Source: CAD feature listing. Evaluate the final solid. Frame: model axes, mm. Face numbers are marked on the shaded views. A direction names the side the tool comes from. Give positions to 0.01 mm unless a question says otherwise; leave off trailing zeros. Write each loop counter-clockwise with the first axis right and the second up, starting at its lowest first coordinate (ties: lowest second). Pieces come first, ordered by that corner, then holes.
```python
from build123d import *

# Parameters (mm, degrees)
SKETCH_2_W                  = 130
SKETCH_2_H                  = 90
EXTRUDE_1_DEPTH             = 110
SKETCH_3_W                  = 124
SKETCH_3_H                  = 107
CUT_EXTRUDE_1_DEPTH         = 87
CUT_EXTRUDE_5_REACH         = 178.139
EXTRUDE_5_DEPTH             = 11
SKETCH_16_W                 = 5.817441426
SKETCH_16_H                 = 7.857396668
CUT_EXTRUDE_6_DEPTH         = 9
FILLET_8_R                  = 3
FILLET_9_R                  = 3
SKETCH_17_W                 = 8
SKETCH_17_H                 = 8
SKETCH_17_R                 = 1.5
EXTRUDE_6_DEPTH             = 6
PATTERN_LINEAR_1_COUNT      = 2
PATTERN_LINEAR_1_PITCH      = 116
PATTERN_LINEAR_1_COUNT_DIR2 = 2
PATTERN_LINEAR_1_PITCH_DIR2 = 76
EXTRUDE_7_DEPTH             = 6
EXTRUDE_8_DEPTH             = 6
SKETCH_20_W                 = 5.7
SKETCH_20_H                 = 2.6
CUT_EXTRUDE_7_DEPTH         = 7.5
PATTERN_LINEAR_2_COUNT      = 2
PATTERN_LINEAR_2_PITCH      = 116
PATTERN_LINEAR_2_COUNT_DIR2 = 2
PATTERN_LINEAR_2_PITCH_DIR2 = 76
SKETCH_23_W                 = 8
SKETCH_23_H                 = 8
SKETCH_23_R                 = 1.55
EXTRUDE_9_DEPTH             = 6
PATTERN_LINEAR_3_COUNT      = 2
PATTERN_LINEAR_3_PITCH      = 116
PATTERN_LINEAR_3_COUNT_DIR2 = 2
PATTERN_LINEAR_3_PITCH_DIR2 = 90
EXTRUDE_10_DEPTH            = 8
EXTRUDE_11_DEPTH            = 8
PATTERN_LINEAR_4_COUNT      = 2
PATTERN_LINEAR_4_PITCH      = 90
PATTERN_LINEAR_5_COUNT      = 2
PATTERN_LINEAR_5_PITCH      = 90
SKETCH_27_W                 = 5.7
SKETCH_27_H                 = 2.6
CUT_EXTRUDE_8_DEPTH         = 7.5
PATTERN_LINEAR_6_COUNT      = 2
PATTERN_LINEAR_6_PITCH      = 116
SKETCH_28_W                 = 5.7
SKETCH_28_H                 = 2.6
CUT_EXTRUDE_9_DEPTH         = 7.5
PATTERN_LINEAR_7_COUNT      = 2
PATTERN_LINEAR_7_PITCH      = 116


with BuildPart() as part:
    # Sketch 2 → Extrude 1 (new body)
    with BuildSketch(Plane.XY):
        Rectangle(SKETCH_2_W, SKETCH_2_H)
    extrude(amount=EXTRUDE_1_DEPTH)

    # Sketch 3 → Cut-Extrude 1 (cut)
    with BuildSketch(Plane(origin=(0, 45, 0), x_dir=(1, 0, 0), z_dir=(0, 1, 0))):
        with Locations((0, -56.5)):
            Rectangle(SKETCH_3_W, SKETCH_3_H)
    extrude(amount=-CUT_EXTRUDE_1_DEPTH, mode=Mode.SUBTRACT)

    # Sketch 13 → Cut-Extrude 5 (cut, up to next)
    with BuildSketch(Plane.ZY.offset(65), mode=Mode.PRIVATE) as cut_extrude_5_sk1:
        Polygon((15, -42), (23, -42), (23, -28.8), (20.505788704, -26.3), (17.494211296, -26.3), (15, -28.8), align=None)
    cut_extrude_5_tool1 = extrude(cut_extrude_5_sk1.sketch, amount=-CUT_EXTRUDE_5_REACH, mode=Mode.PRIVATE) & part.part
    add(cut_extrude_5_tool1.solids().sort_by_distance((-65, -34.516546, 19))[0], mode=Mode.SUBTRACT)

    # Sketch 15 → Extrude 5 (add)
    with BuildSketch(Plane(origin=(0, -42, 0), x_dir=(1, 0, 0), z_dir=(0, 1, 0))):
        Polygon((-62, -25), (-46.7, -25), (-46.7, -13), (-62, -13), (-62, -15), (-48.7, -15), (-48.7, -23), (-62, -23), align=None)
    extrude(amount=EXTRUDE_5_DEPTH)

    # Sketch 16 → Cut-Extrude 6 (cut)
    with BuildSketch(Plane(origin=(0, -31, 0), x_dir=(1, 0, 0), z_dir=(0, 1, 0))):
        with Locations((-46.7, -19)):
            Rectangle(SKETCH_16_W, SKETCH_16_H)
    extrude(amount=-CUT_EXTRUDE_6_DEPTH, mode=Mode.SUBTRACT)

    # Fillet 8
    fillet_8_edges = [part.edges().sort_by_distance(p)[0] for p in [
        (-65, 0, 0),
    ]]
    fillet(fillet_8_edges, radius=FILLET_8_R)

    # Fillet 9
    fillet_9_edges = [part.edges().sort_by_distance(p)[0] for p in [
        (65, 0, 0),
    ]]
    fillet(fillet_9_edges, radius=FILLET_9_R)

    # Sketch 17 → Extrude 6 (add)
    with BuildSketch(Plane.XY.offset(110)):
        with Locations((-58, -38)):
            Rectangle(SKETCH_17_W, SKETCH_17_H)
        with Locations((-58, -38)):
            Circle(SKETCH_17_R, mode=Mode.SUBTRACT)
    extrude_6 = extrude(amount=-EXTRUDE_6_DEPTH)

    # Pattern Linear 1: Extrude 6 2 × 2
    with Locations(*[(i * PATTERN_LINEAR_1_PITCH, j * PATTERN_LINEAR_1_PITCH_DIR2, 0) for i in range(PATTERN_LINEAR_1_COUNT) for j in range(PATTERN_LINEAR_1_COUNT_DIR2) if (i, j) != (0, 0)]):
        add(extrude_6)

    # Sketch 18 → Extrude 7 (add)
    with BuildSketch(Plane.XY.offset(110)):
        Polygon((-54, 34), (-62, 34), (-62, 26), align=None)
    extrude(amount=-EXTRUDE_7_DEPTH)

    # Sketch 19 → Extrude 8 (add)
    with BuildSketch(Plane.XY.offset(110)):
        Polygon((62, 34), (54, 34), (62, 26), align=None)
    extrude(amount=-EXTRUDE_8_DEPTH)

    # Sketch 20 → Cut-Extrude 7 (cut)
    with BuildSketch(Plane(origin=(0, -34, 0), x_dir=(1, 0, 0), z_dir=(0, 1, 0))):
        with Locations((-58, -107)):
            Rectangle(SKETCH_20_W, SKETCH_20_H)
    cut_extrude_7 = extrude(amount=-CUT_EXTRUDE_7_DEPTH, mode=Mode.SUBTRACT)

    # Pattern Linear 2: Cut-Extrude 7 2 × 2
    with Locations(*[(i * PATTERN_LINEAR_2_PITCH, j * PATTERN_LINEAR_2_PITCH_DIR2, 0) for i in range(PATTERN_LINEAR_2_COUNT) for j in range(PATTERN_LINEAR_2_COUNT_DIR2) if (i, j) != (0, 0)]):
        add(cut_extrude_7, mode=Mode.SUBTRACT)



with BuildPart() as body_2:
    # Sketch 23 → Extrude 9 (new body)
    with BuildSketch(Plane(origin=(0, 45, 0), x_dir=(1, 0, 0), z_dir=(0, 1, 0))):
        with Locations((-58, -7)):
            Rectangle(SKETCH_23_W, SKETCH_23_H)
        with Locations(Location((-58, -7, 0), (0, 0, 270))):
            Circle(SKETCH_23_R, mode=Mode.SUBTRACT)
    extrude_9 = extrude(amount=-EXTRUDE_9_DEPTH)


with BuildPart() as pattern_linear_3_1:
    # Pattern Linear 3: pattern copy
    add(extrude_9.moved(Location(Vector(1, 0, 0) * (0 * PATTERN_LINEAR_3_PITCH) + Vector(0, 0, 1) * (1 * PATTERN_LINEAR_3_PITCH_DIR2))))


with BuildPart() as pattern_linear_3_2:
    # Pattern Linear 3: pattern copy
    add(extrude_9.moved(Location(Vector(1, 0, 0) * (1 * PATTERN_LINEAR_3_PITCH) + Vector(0, 0, 1) * (0 * PATTERN_LINEAR_3_PITCH_DIR2))))


with BuildPart() as pattern_linear_3_3:
    # Pattern Linear 3: pattern copy
    add(extrude_9.moved(Location(Vector(1, 0, 0) * (1 * PATTERN_LINEAR_3_PITCH) + Vector(0, 0, 1) * (1 * PATTERN_LINEAR_3_PITCH_DIR2))))


with BuildPart() as part_1:
    add(part.part)

    add(body_2.part)  # Extrude 10 merges body 2
    # Sketch 24 → Extrude 10 (add)
    with BuildSketch(Plane.XY.offset(3)):
        Polygon((-54, 39), (-62, 39), (-62, 31), align=None)
    extrude_10 = extrude(amount=EXTRUDE_10_DEPTH)


    add(pattern_linear_3_2.part)  # Extrude 11 merges Pattern Linear 3_2
    # Sketch 25 → Extrude 11 (add)
    with BuildSketch(Plane.XY.offset(3)):
        Polygon((54, 39), (62, 39), (62, 31), align=None)
    extrude_11 = extrude(amount=EXTRUDE_11_DEPTH)


    add(pattern_linear_3_1.part)  # Pattern Linear 4 merges Pattern Linear 3_1
    # Pattern Linear 4: Extrude 10 ×2
    with Locations(*[(0, 0, i * PATTERN_LINEAR_4_PITCH) for i in range(1, PATTERN_LINEAR_4_COUNT)]):
        add(extrude_10)


    add(pattern_linear_3_3.part)  # Pattern Linear 5 merges Pattern Linear 3_3
    # Pattern Linear 5: Extrude 11 ×2
    with Locations(*[(0, 0, i * PATTERN_LINEAR_5_PITCH) for i in range(1, PATTERN_LINEAR_5_COUNT)]):
        add(extrude_11)

    # Sketch 27 → Cut-Extrude 8 (cut)
    with BuildSketch(Plane.XY.offset(11)):
        with Locations((-58, 42.036350265)):
            Rectangle(SKETCH_27_W, SKETCH_27_H)
    cut_extrude_8 = extrude(amount=-CUT_EXTRUDE_8_DEPTH, mode=Mode.SUBTRACT)

    # Pattern Linear 6: Cut-Extrude 8 ×2
    with Locations(*[(i * PATTERN_LINEAR_6_PITCH, 0, 0) for i in range(1, PATTERN_LINEAR_6_COUNT)]):
        add(cut_extrude_8, mode=Mode.SUBTRACT)

    # Sketch 28 → Cut-Extrude 9 (cut)
    with BuildSketch(Plane(origin=(0, 0, 93), x_dir=(-1, 0, 0), z_dir=(0, 0, -1))):
        with Locations((-58, 42)):
            Rectangle(SKETCH_28_W, SKETCH_28_H)
    cut_extrude_9 = extrude(amount=-CUT_EXTRUDE_9_DEPTH, mode=Mode.SUBTRACT)

    # Pattern Linear 7: Cut-Extrude 9 ×2
    with Locations(*[(-i * PATTERN_LINEAR_7_PITCH, 0, 0) for i in range(1, PATTERN_LINEAR_7_COUNT)]):
        add(cut_extrude_9, mode=Mode.SUBTRACT)


solid = part_1.part
```
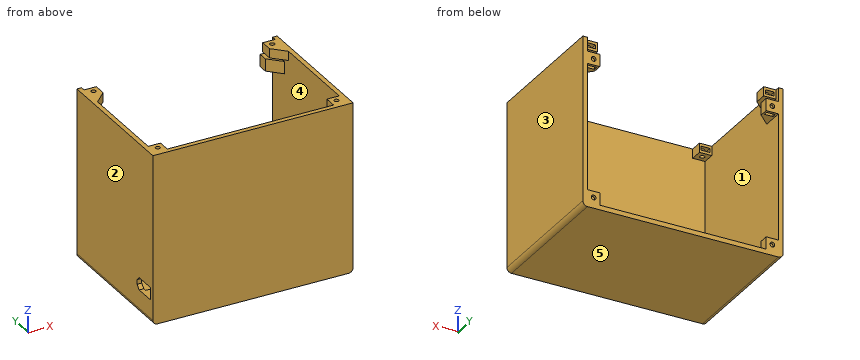
1. Line query: probe 1 along X at (y, z) = (44.65, 7); probe 2 along X at (y, z) = (9, 56); probe 3 along Y at (x, z) = (57, 73). Output: solid intervals per line, ascending.
2. Section query A-A (y = -23.5). Return loops of the section in (x, z), plus the area to 3 significant figures.
3. Pull-direction query (Z, two-part tool) for the marked faces 3, 4 and 5; classes: pulls with the +Z half, pulls with the -Z half, needs draft (parallel to the pull), parting line crosses it, or undercut.
4. Access query for the marked faces 1 and 2. Directions: +Z, -Z, +X, -X, +Y, -Y. A direction counts if a zero-diameter tool reaches every point of the face in a straight line with its end or side. Return the directions, or none.
5. Pin query (flat end, axial travel): P1, Ø8, axis at x = -36.5, y = 14.5, coming from the +Z side; P2, Ø5, axis at x = -58, z = 7, coming from the +Y side; P3, Ø4, axis at x = -53, z = 18.5, coming from the +Y side; P4, Ø0.8, axis at x = -58, z = 106.5, coming from the +Y side. Return the tip coordinate at first contact, or that it passes through.
6. Section query C-C (z = 55.5). Return loops of the section in (x, y), plus the area to 3 significant figures.
7. Section query B-B (x = 52). Return loops of the section in (y, z).
The answers:
1. probe 1: x = -65 to -59.55, -56.45 to -54, 54 to 56.45, 59.55 to 65
1. probe 2: x = -65 to -62, 62 to 65
1. probe 3: y = -45 to -42
2. outline: (-65, 3) arc R3 ccw to (-62, 0) - (62, 0) arc R3 ccw to (65, 3) - (65, 110) - (62, 110) - (62, 3) - (-62, 3) - (-62, 110) - (-65, 110) - close
2. area: 1,030 mm2
3. face 3: needs draft
3. face 4: undercut
3. face 5: pulls with the -Z half
4. face 1: none
4. face 2: +Z, -Z, -X, +Y, -Y
5. P1: stops at z = 3
5. P2: stops at y = 45
5. P3: stops at y = -42
5. P4: stops at y = 34.5
6. outline: (-65, -45) - (65, -45) - (65, 45) - (62, 45) - (62, -42) - (-62, -42) - (-62, 45) - (-65, 45) - close
6. area: 912 mm2
7. outline: (-45, 0) - (45, 0) - (45, 3) - (-42, 3) - (-42, 110) - (-45, 110) - close
